Build history of the part. All positions in model axes, mm. A direction names the side the tool comes from. Round coordinates to 2 decimals unless told otherwise and drop trailing zeros. Write each loop counter-clockwise with the first axis right and the second up, starting at its lowest first coordinate (ties: lowest second). Pieces come first, ordered by that corner, then holes. Notation, with made-up numbers: (75.25, -4.5) -> (90.25, -4.5) arc R25 cw to (90.25, 13.5) -> close; hole circle Ø9 at (-30.75, -32). An arc over 180 degrees is marked (long way). Return JSON: item names as keys, results as strings.
from build123d import *

# Parameters (mm, degrees)
SKETCH003_R     = 30
PAD001_DEPTH    = 2
SKETCH012_R     = 1.75
POCKET005_DEPTH = 5
SKETCH024_W     = 25
SKETCH024_H     = 3.5
SKETCH024_W_2   = 20
POCKET016_DEPTH = 5


with BuildPart() as part:
    # Sketch003 → Pad001 (new body)
    with BuildSketch(Plane.XY):
        Circle(SKETCH003_R)
    extrude(amount=PAD001_DEPTH)

    # Sketch012 (on Face3 of Pad001) → Pocket005 (cut)
    with BuildSketch(Plane.XY.offset(2)):
        with Locations((14.520833, 19.108778)):
            Circle(SKETCH012_R)
        with Locations((-24, 0)):
            Circle(SKETCH012_R)
        with Locations((14.520833, -19.108778)):
            Circle(SKETCH012_R)
    extrude(amount=-POCKET005_DEPTH, mode=Mode.SUBTRACT)

    # Sketch024 (on Face3 of Pocket005) → Pocket016 (cut)
    with BuildSketch(Plane.XY.offset(2)):
        with Locations((3.5, 10.25)):
            Rectangle(SKETCH024_W, SKETCH024_H)
        with Locations((6, -10.25)):
            Rectangle(SKETCH024_W_2, SKETCH024_H)
    extrude(amount=-POCKET016_DEPTH, mode=Mode.SUBTRACT)


with BuildPart() as part_1:
    # Body001 placement: moved
    add(part.part.moved(Location((0, 0, 26))))


solid = part_1.part
Q1. Saw through at B-B on x = 0. List the corners of the cut face in (y, z).
Verdict:
{"outline": "(-30, 26) -> (-12, 26) -> (-12, 28) -> (-30, 28) -> close; (-8.5, 26) -> (8.5, 26) -> (8.5, 28) -> (-8.5, 28) -> close; (12, 26) -> (30, 26) -> (30, 28) -> (12, 28) -> close"}
Q2. Saw through at A-A on y = 0. List the corners of the cut face in (x, z).
Verdict:
{"outline": "(-30, 26) -> (-25.75, 26) -> (-25.75, 28) -> (-30, 28) -> close; (-22.25, 26) -> (30, 26) -> (30, 28) -> (-22.25, 28) -> close"}
Q3. Saw through at D-D on z = 27.4. List the corners of the cut face in (x, y).
Verdict:
{"outline": "circle Ø60 at (0, 0); hole circle Ø3.5 at (-24, 0); hole (-9, 8.5) -> (16, 8.5) -> (16, 12) -> (-9, 12) -> close; hole (-4, -12) -> (16, -12) -> (16, -8.5) -> (-4, -8.5) -> close; hole circle Ø3.5 at (14.52, -19.11); hole circle Ø3.5 at (14.52, 19.11)"}
Q4. Wall check: L1, parallel to Y at x = 6, z = 26.3; L2, parallel to Y at x = 13, z = 27.9; L3, parallel to Y at x = -1.5, z = 27.05. Give the ranges that are in metal, low to high.
Verdict:
{"L1": "y = -29.39 to -12, -8.5 to 8.5, 12 to 29.39", "L2": "y = -27.04 to -19.97, -18.24 to -12, -8.5 to 8.5, 12 to 18.24, 19.97 to 27.04", "L3": "y = -29.96 to -12, -8.5 to 8.5, 12 to 29.96"}
Q5. Pin check, flat tips, straight feed: pin 1 Ø1 at (x, z) = (2, 26.5) entering from -Y; pin 2 Ø0.6 at (x, z) = (-1, 27) entering from +Y; pin 3 Ø1 at (x, z) = (7.5, 26.5) entering from +Y; pin 4 Ø3 at (x, y) = (-24, 0) entering from -Z. Stop position of each tip, or through.
Verdict:
{"pin 1": "stops at y = -29.96", "pin 2": "stops at y = 29.99", "pin 3": "stops at y = 29.17", "pin 4": "passes through"}
Q6. Saw through at C-C on x = -24. List the corners of the cut face in (y, z).
Verdict:
{"outline": "(-18, 26) -> (-1.75, 26) -> (-1.75, 28) -> (-18, 28) -> close; (1.75, 26) -> (18, 26) -> (18, 28) -> (1.75, 28) -> close"}
Q7. Two-plate mould, pull along Y, no slides. Class faces 3 (the flat face through (6, -12, 27)), 4 (the cylindrical face through (-29.97, 1.32, 26.99)), 5 (the flat face through (0, 0, 28)): +Y half, -Y half, draft (parallel to the pull), parting line (faces both ways), or undercut.
Verdict:
{"face 3": "undercut", "face 4": "parting line", "face 5": "draft"}
Q8. 3-axis set-ups, long thin cutter, end or side, ignore diameter. For faces 1 (the flat face through (0, 0, 26)), 2 (the flat face through (-4, -10, 27)): which of +Z, -Z, +X, -X, +Y, -Y reach the whole face in a straight line?
Verdict:
{"face 1": "-Z, +X, -X, +Y, -Y", "face 2": "+Z, -Z"}
